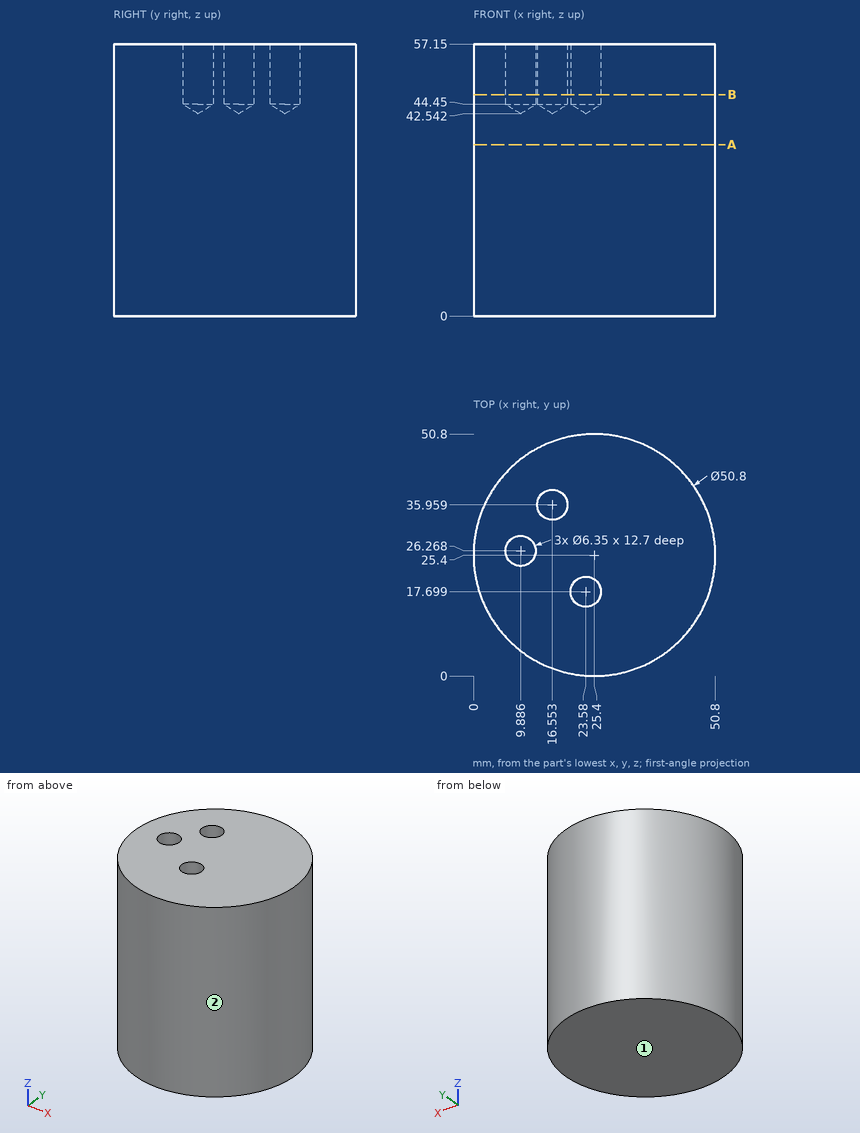
Geometry: see drawing. Coordinates: mm, zero at the bounding-box minimum. Round coordinates to 2 decimals unless told otherwise and drop trailing zeros. Loops run counter-clockwise (first coordinate to the right, second up) from the corner with the lowest first, then second, coordinate; pieces in that order, holes last. Notation, with made-up numbers: M -26,4 L 15,4 A20 cw 15,23 Z; hole C 86,9 d5. An arc over 180 degrees is marked long. Use a Markdown table: item, result. Add a question column.
1. Section query B-B on z = 46.5. Give the number of separate pieces and of enclosed holes in the cut face, then the cut area to 3 significant figures.
2. Section query A-A on z = 36. Return the cut outline in (x, y).
3. Line query: line 1 (X direction, y = 25.5, z = 50) (1 decimal); line 2 (Y direction, x = 17, z = 54) (1 decimal); line 3 (X direction, y = 9, z = 38) (1 decimal). Output: solid intervals per line, ascending.
4. Contact query for flat-ended pins moving along their axis: P1, Ø3, axis at y = 14, z = 42, coming from the -X side; P2, Ø5, axis at x = 15.5, z = 36, coming from the +Y side; P3, Ø1, axis at x = 21, z = 46, coming from the -Y side; P4, Ø5, axis at x = 23.58, y = 17.7, coming from the -Z side. Output: stop coordinate, or through.
5. Mould query, pull axis Y, two halves, no side actions, for the marked faces 1 and 2. Classes: pulls with the +Y half, pulls with the -Y half, needs draft (parallel to the pull), parting line crosses it, or undercut.
Reported:
| question | item | result |
|---|---|---|
| 1 | separate pieces | 1 |
| 1 | enclosed holes | 3 |
| 1 | area | 1,930 mm² |
| 2 | outline | C 25.4,25.4 d50.8 |
| 3 | line 1 | x = 0 to 6.8, 13 to 50.8 |
| 3 | line 2 | y = 1.4 to 32.8, 39.1 to 49.4 |
| 3 | line 3 | x = 6 to 44.8 |
| 4 | P1 | stops at x = 2.01 |
| 4 | P2 | stops at y = 49.7 |
| 4 | P3 | stops at y = 0.3 |
| 4 | P4 | stops at z = 0 |
| 5 | face 1 | needs draft |
| 5 | face 2 | parting line crosses it |
